Check sheet for the drawn part. Datum: minimum x, y, z corner. Units: mm. A direction names the side the tool comes from. Give positions to 0.01 mm unless a question says otherwise; leave off trailing zeros. Loops run counter-clockwise (first coordinate to the right, second up) from the corner with the lowest first, then second, coordinate; pieces in that order, holes last. Notation, with made-up numbers: (81, 53.5) - (121, 53.5) arc R26 cw to (121, 71.5) - close; hole circle Ø1 at (63, 43.5). An arc over 180 degrees is marked (long way). Use one line per item in the form item = value.
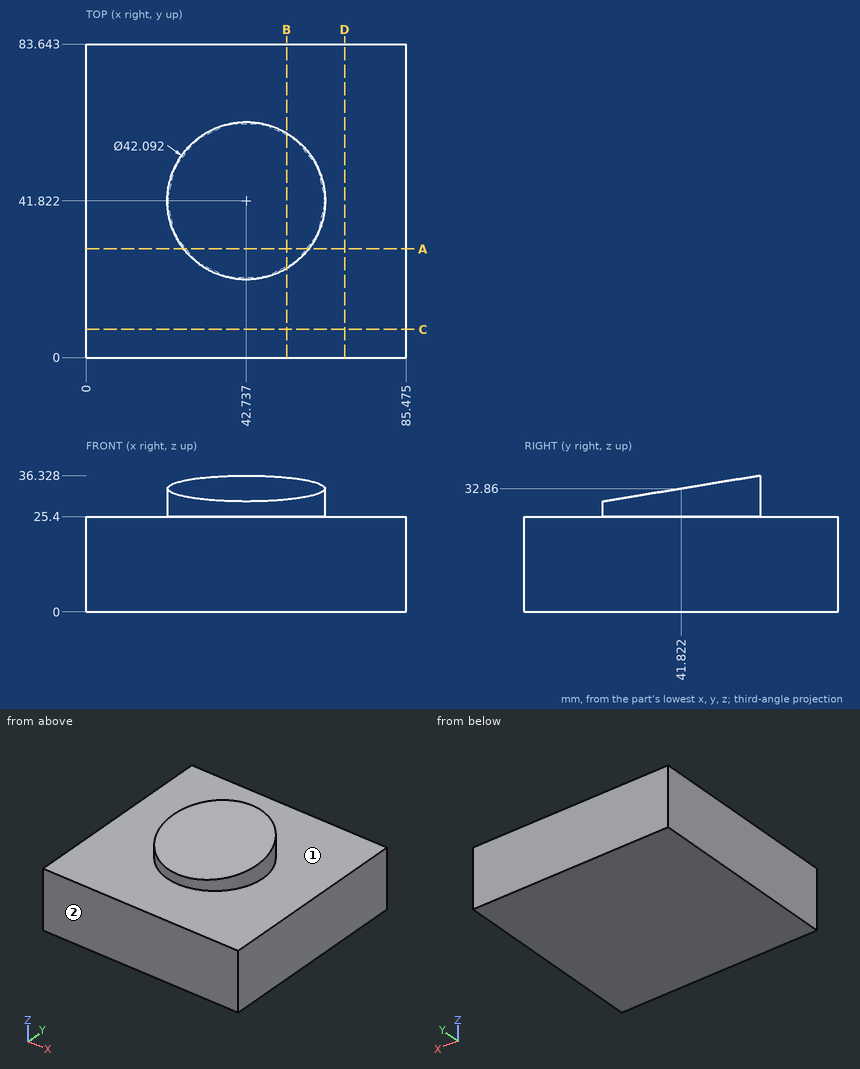
1. Section check B-B, the plane x = 53.5. Record the cut outline in (y, z).
Result set:
outline = (0, 0) - (83.64, 0) - (83.64, 25.4) - (59.91, 25.4) - (59.91, 35.84) - (23.74, 29.88) - (23.74, 25.4) - (0, 25.4) - close
2. Section check C-C, the plane y = 7.5. Record the cut outline in (x, z) (1 decimal), then the cut area to 3 significant figures.
Result set:
outline = (0, 0) - (85.5, 0) - (85.5, 25.4) - (0, 25.4) - close
area = 2,170 mm²
3. Section check D-D, the plane x = 69. Record the cut outline in (y, z), then the cut area to 3 significant figures.
Result set:
outline = (0, 0) - (83.64, 0) - (83.64, 25.4) - (0, 25.4) - close
area = 2,120 mm²
4. Depth check by flat-ended pin: pin 1 Ø2 at (x, y) = (11, 23) entering from +Z; pin 2 Ø25 at (x, y) = (44.5, 39) entering from +Z (1 decimal); pin 3 Ø1.5 at (x, z) = (50, 27.5) entering from -Y. Enter the tip coordinate at first touch or a pass-through.
Result set:
pin_1 = 25.4
pin_2 = 34.5
pin_3 = 21.81
5. Section check A-A, the plane y = 29. Record the cut outline in (x, z) (1 decimal), then the cut area to 3 significant figures.
Result set:
outline = (0, 0) - (85.5, 0) - (85.5, 25.4) - (59.4, 25.4) - (59.4, 30.7) - (26, 30.7) - (26, 25.4) - (0, 25.4) - close
area = 2,350 mm²
6. Tool access check on the marked faces 1 and 2. Record the directions out of +Z, -Z, +X, -X, +Y, -Y that give a thin tool (end or side, any length) a straight path to the whole face; none if there is none.
Result set:
face_1 = +Z
face_2 = +Z, -Z, +X, -X, -Y
7. Scan lines: probe 1 along Z at (x, y) = (67.5, 22); probe 2 along X at (y, z) = (29.5, 26) (1 decimal); probe 3 along Z at (x, y) = (44, 50). Record each from-to range of solid material in increasing order.
Result set:
probe_1 = 0 to 25.4
probe_2 = 25.7 to 59.8
probe_3 = 0 to 34.21
